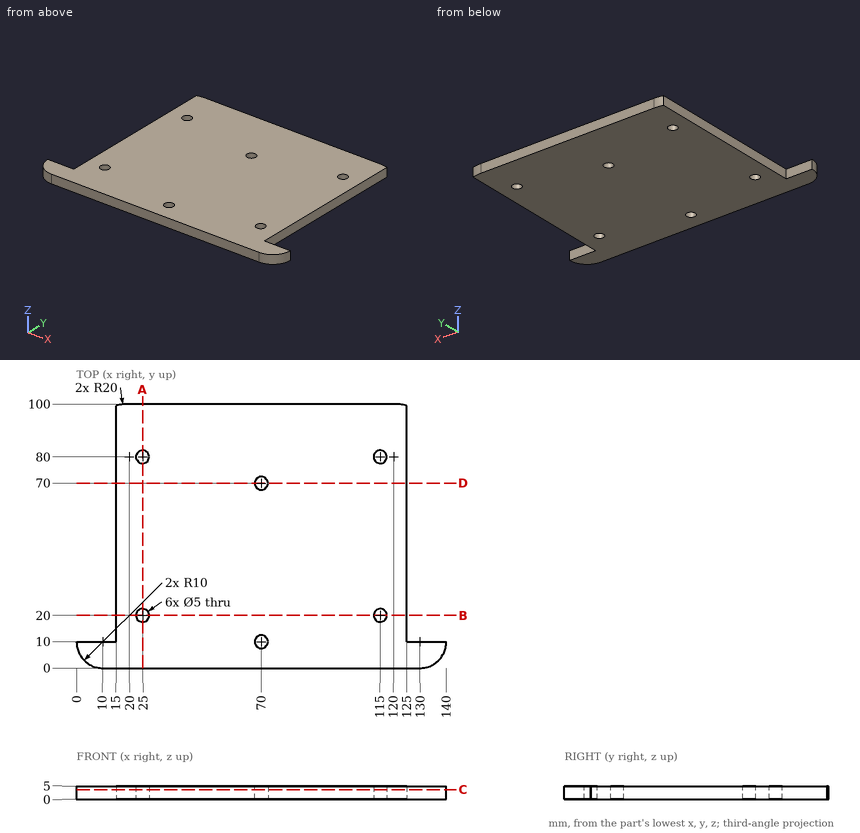
Answer from the drawing. Dimensions are ordinates in mm from the lowest x, y and z of the part. Coordinates: 2 decimals unless noted, no trailing zeros. Loops run counter-clockwise (first coordinate to the right, second up) from the corner with the lowest first, then second, coordinate; pieces in that order, holes last.
1) Section A-A (x = 25) is taken. Give the vertices of the cut face in (y, z).
Results:
outline: (0, 0) - (17.5, 0) - (17.5, 5) - (0, 5) - close; (22.5, 0) - (77.5, 0) - (77.5, 5) - (22.5, 5) - close; (82.5, 0) - (100, 0) - (100, 5) - (82.5, 5) - close
2) Flat-ended cylindrical pins translate along their axes: pin 1 (1 mm diameter, centred on y = 26.5, z = 0.5, fed in from -X); pin 2 (2.5 mm diameter, centred on x = 4, z = 2, fed in from +Y); pin 3 (1 mm diameter, centred on y = 80, z = 1, fed in from +X). Find the tip coordinate at first contact, or state that the pin passes through.
Results:
pin 1: stops at x = 15
pin 2: stops at y = 10
pin 3: stops at x = 125
3) Section D-D (y = 70) is taken. Give the vertices of the cut face in (x, z), plus the area to 3 significant figures.
Results:
outline: (15, 0) - (67.5, 0) - (67.5, 5) - (15, 5) - close; (72.5, 0) - (125, 0) - (125, 5) - (72.5, 5) - close
area: 525 mm2
4) Section C-C (z = 3.65) is taken. Give the vertices of the cut face in (x, y).
Results:
outline: (0, 10) arc R10 ccw to (10, 0) - (130, 0) arc R10 ccw to (140, 10) - (125, 10) - (125, 99.36) arc R20 ccw to (120, 100) - (20, 100) arc R20 ccw to (15, 99.36) - (15, 10) - close; hole circle Ø5 at (25, 20); hole circle Ø5 at (25, 80); hole circle Ø5 at (70, 10); hole circle Ø5 at (70, 70); hole circle Ø5 at (115, 20); hole circle Ø5 at (115, 80)
5) Consider probe 1 along Y at (x, z) = (70, 2.8); probe 2 along Y at (x, z) = (25, 3.8); probe 3 along X at (y, z) = (59.5, 0.9). Determine where each line is inside the solid, lowest interval first.
Results:
probe 1: y = 0 to 7.5, 12.5 to 67.5, 72.5 to 100
probe 2: y = 0 to 17.5, 22.5 to 77.5, 82.5 to 100
probe 3: x = 15 to 125
6) Section B-B (y = 20) is taken. Give the vertices of the cut face in (x, z), plus the area to 3 significant figures.
Results:
outline: (15, 0) - (22.5, 0) - (22.5, 5) - (15, 5) - close; (27.5, 0) - (112.5, 0) - (112.5, 5) - (27.5, 5) - close; (117.5, 0) - (125, 0) - (125, 5) - (117.5, 5) - close
area: 500 mm2
